Geometry check sheet. Reference: the model listing, model coordinates, mm. Face numbers are marked on the shaded views. A direction names the side the tool comes from. Round coordinates to 2 decimals unless told otherwise and drop trailing zeros. Write each loop counter-clockwise with the first axis right and the second up, starting at its lowest first coordinate (ties: lowest second). Pieces come first, ordered by that corner, then holes. Notation, with made-up numbers: M 59.5,-25 L 117.5,-25 A26 ccw 117.5,11 Z; hole C 48,63 d6. An arc over 180 degrees is marked long. Put each result on its own line as item: value. Start each with the question number.
(1) Gauge pin test, flat ends, axial feed: pin 1 (1.3 mm diameter, centred on y = 0.5, z = 1.5, fed in from -X); pin 2 (1.5 mm diameter, centred on x = -7.5, z = 11, fed in from +Y); pin 3 (1.3 mm diameter, centred on x = 2.5, z = 0.5, fed in from -Y). Record the tip position at first contact, or that the pin passes through.
(2) Section check B-B on x = 0. Record the cut outline in (y, z), then the cut area to 3 significant figures.
(3) Section check A-A on x = -4.5. Record the cut outline in (y, z).
(4) Mould release check, pull along Z, two halves, no side actions. Record for the marked faces 5, 6 and 7: pulls with the +Z half, pulls with the -Z half, needs draft (parallel to the pull), parting line crosses it, or undercut.
(5) Material ranges on probe 1 along X at (y, z) = (-15, 6.25); probe 2 along X at (y, z) = (4.5, 2); probe 3 along Y at (x, z) = (2, 6.75), recorded low to high.
(6) Tool access check on the marked faces 1, 2, 3 and 4. Record the directions out of +Z, -Z, +X, -X, +Y, -Y that give a thin tool (end or side, any length) a straight path to the whole face; none if there is none.
(7) Section check C-C on z = 1.5. Record the cut outline in (x, y).
(8) Section check D-D on y = 0. Record the cut outline in (x, z), then the cut area to 3 significant figures.
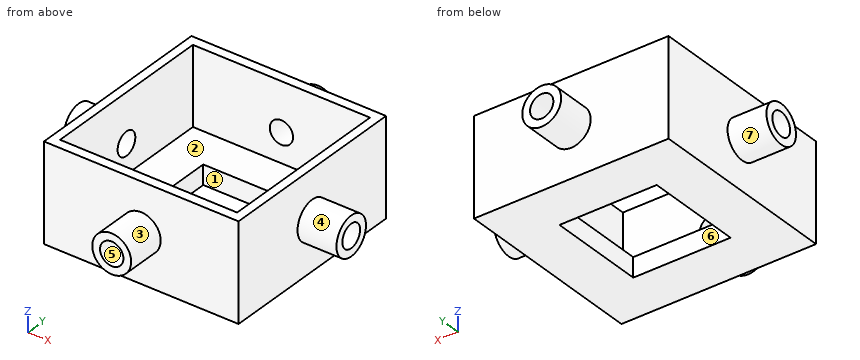
from build123d import *

# Parameters (mm, degrees)
F0_W      = 25.4
F0_H      = 25.4
F1_DEPTH  = 12.7
F2_W      = 23.1146477163
F2_H      = 22.8712297976
F3_DEPTH  = 10.16
F4_R      = 2.54
F5_DEPTH  = 5.08
F6_R      = 2.54
F7_DEPTH  = 5.08
F8_R      = 1.524
F9_DEPTH  = 35.561
F10_R     = 2.54
F11_DEPTH = 5.08
F12_R     = 2.54
F13_DEPTH = 5.08
F14_R     = 1.524
F15_DEPTH = 35.561
F16_W     = 12.7
F16_H     = 12.7
F17_DEPTH = 2.541


with BuildPart() as f1:
    # F0 (on Top) → F1 (new body)
    with BuildSketch(Plane.XY):
        Rectangle(F0_W, F0_H)
    extrude(amount=F1_DEPTH)

    # F2 (on face) → F3 (cut)
    with BuildSketch(Plane.XY.offset(12.7)):
        Rectangle(F2_W, F2_H)
    extrude(amount=-F3_DEPTH, mode=Mode.SUBTRACT)

    # F4 (on face) → F5 (join)
    with BuildSketch(Plane(origin=(0, 12.7, 0), x_dir=(-1, 0, 0), z_dir=(0, 1, 0))):
        with Locations((0, 6.35)):
            Circle(F4_R)
    extrude(amount=F5_DEPTH)

    # F6 (on face) → F7 (join)
    with BuildSketch(Plane.XZ.offset(12.7)):
        with Locations((0, 6.35)):
            Circle(F6_R)
    extrude(amount=F7_DEPTH)

    # F8 (on face) → F9 (cut, through all)
    with BuildSketch(Plane.XZ.offset(17.78)):
        with Locations((0, 6.35)):
            Circle(F8_R)
    extrude(amount=-F9_DEPTH, mode=Mode.SUBTRACT)

    # F10 (on face) → F11 (join)
    with BuildSketch(Plane.YZ.offset(12.7)):
        with Locations((0, 6.35)):
            Circle(F10_R)
    extrude(amount=F11_DEPTH)

    # F12 (on face) → F13 (join)
    with BuildSketch(Plane(origin=(-12.7, 0, 0), x_dir=(0, -1, 0), z_dir=(-1, 0, 0))):
        with Locations((0, 6.35)):
            Circle(F12_R)
    extrude(amount=F13_DEPTH)

    # F14 (on face) → F15 (cut, through all)
    with BuildSketch(Plane(origin=(-17.78, 0, 0), x_dir=(0, -1, 0), z_dir=(-1, 0, 0))):
        with Locations((0, 6.35)):
            Circle(F14_R)
    extrude(amount=-F15_DEPTH, mode=Mode.SUBTRACT)

    # F16 (on face) → F17 (cut, through all)
    with BuildSketch(Plane.XY.offset(2.54)):
        Rectangle(F16_W, F16_H)
    extrude(amount=-F17_DEPTH, mode=Mode.SUBTRACT)


solid = f1.part
Answers follow:
1. pin 1: stops at x = -12.7
1. pin 2: stops at y = 12.7
1. pin 3: stops at y = -12.7
2. outline: M -17.78,3.81 L -12.7,3.81 L -12.7,0 L -6.35,0 L -6.35,2.54 L -11.44,2.54 L -11.44,4.83 L -17.78,4.83 Z; M -17.78,7.87 L -11.44,7.87 L -11.44,12.7 L -12.7,12.7 L -12.7,8.89 L -17.78,8.89 Z; M 6.35,0 L 12.7,0 L 12.7,3.81 L 17.78,3.81 L 17.78,4.83 L 11.44,4.83 L 11.44,2.54 L 6.35,2.54 Z; M 11.44,7.87 L 17.78,7.87 L 17.78,8.89 L 12.7,8.89 L 12.7,12.7 L 11.44,12.7 Z
2. area: 70.9 mm^2
3. outline: M -12.7,0 L -6.35,0 L -6.35,2.54 L -11.44,2.54 L -11.44,12.7 L -12.7,12.7 Z; M 6.35,0 L 12.7,0 L 12.7,12.7 L 11.44,12.7 L 11.44,2.54 L 6.35,2.54 Z
4. face 5: undercut
4. face 6: needs draft
4. face 7: parting line crosses it
5. probe 1: x = -2.54 to -1.52, 1.52 to 2.54
5. probe 2: x = -12.7 to -6.35, 6.35 to 12.7
5. probe 3: y = -17.78 to -11.44, 11.44 to 17.78
6. face 1: +Z, -Z
6. face 2: +Z
6. face 3: -Y
6. face 4: +X
7. outline: M -12.7,-12.7 L 12.7,-12.7 L 12.7,12.7 L -12.7,12.7 Z; hole M -6.35,-6.35 L 6.35,-6.35 L 6.35,6.35 L -6.35,6.35 Z
8. outline: M -17.78,3.81 L -12.7,3.81 L -12.7,0 L -6.35,0 L -6.35,2.54 L -11.56,2.54 L -11.56,4.83 L -17.78,4.83 Z; M -17.78,7.87 L -11.56,7.87 L -11.56,12.7 L -12.7,12.7 L -12.7,8.89 L -17.78,8.89 Z; M 6.35,0 L 12.7,0 L 12.7,3.81 L 17.78,3.81 L 17.78,4.83 L 11.56,4.83 L 11.56,2.54 L 6.35,2.54 Z; M 11.56,7.87 L 17.78,7.87 L 17.78,8.89 L 12.7,8.89 L 12.7,12.7 L 11.56,12.7 Z
8. area: 69.2 mm^2
